from build123d import *

# Parameters (mm, degrees)
F0_R           = 10
F0_R_2         = 6.3
F1_DEPTH       = 6
F2_DEPTH       = 15
F4_R           = 1
F1_FACE_R      = 10
F7_D           = 4.3
F7_CBORE_D     = 8
F7_CBORE_DEPTH = 4.2
F8_D           = 3.2
F8_DEPTH       = 8
F8_START       = 6
F8_TIP         = 0.9613769904


with BuildPart() as f1:
    # F0 (on Top) → F1 (new body)
    with BuildSketch(Plane.XY):
        Circle(F0_R)
        Circle(F0_R_2, mode=Mode.SUBTRACT)
        Circle(F0_R_2)
    extrude(amount=F1_DEPTH)

    # F0 (on Top) → F2 (join)
    with BuildSketch(Plane.XY):
        Circle(F0_R)
        Circle(F0_R_2, mode=Mode.SUBTRACT)
    extrude(amount=-F2_DEPTH)

    # F7 (through all)
    with Locations(Plane(origin=(0, 0, 0), x_dir=(1, 0, 0), z_dir=(0, 0, -1))):
        with Locations((0, 0)):
            CounterBoreHole(F7_D / 2, F7_CBORE_D / 2, F7_CBORE_DEPTH)


with BuildPart() as f5:
    # F4 (on offset) → F5 section 0
    with BuildSketch(Plane.XY.offset(16)):
        Circle(F4_R)
    # F1_face (on face) → F5 section 1
    with BuildSketch(Plane.XY.offset(6)):
        Circle(F1_FACE_R)
    loft()

    # F8
    # its depths count from where the whole tool has entered the part; down to there all is cleared
    with Locations(Plane(origin=(0, 0, 0), x_dir=(1, 0, 0), z_dir=(0, 0, -1)).offset(-F8_START)):
        with Locations((0, 0)):
            Hole(F8_D / 2, depth=F8_DEPTH)
            with Locations((0, 0, -(F8_DEPTH + F8_TIP / 2))):  # 118° drill point
                Cone(0, F8_D / 2, F8_TIP, mode=Mode.SUBTRACT)


solid = f1.part
Can you work these out from the model? Positions are in its coordinate system, mm. A direction names the side the tool comes from. Give positions to 0.01 mm unless a question says otherwise; leave off trailing zeros. Loops run counter-clockwise (first coordinate to the right, second up) from the corner with the lowest first, then second, coordinate; pieces in that order, holes last. Notation, with made-up numbers: (-27, 10) -> (23, 10) arc R9 ccw to (23, 27) -> close; hole circle Ø2 at (28.5, 86.25). An arc over 180 degrees is marked (long way). Write item = value, one per line.
1) Suppose I cut it at C-C on x = 2.75. Write out the boundary of the cut face in (y, z).
Check result:
outline = (-9.61, -15) -> (-5.67, -15) -> (-5.67, 0) -> (-2.9, 0) -> (-2.9, 4.2) -> (2.9, 4.2) -> (2.9, 0) -> (5.67, 0) -> (5.67, -15) -> (9.61, -15) -> (9.61, 6) -> (-9.61, 6) -> close
2) Thinking about a two-plate mould opening in Y: for faces 3 (the flat face through (4.1, -1.3, 0)), 4 (the cylindrical face through (-2.17, -9.76, -4.35)), 5 (the flat face through (-0.1, 2.4, 6)), which applies, released by +Y, released by -Y, zero draft, split by the parting line, or undercut?
Check result:
face_3 = undercut
face_4 = split by the parting line
face_5 = zero draft
3) For faces 1 (the cylindrical face through (2.15, -0.09, 5.11)), 2 (the flat face through (2, 2, 4.2)), which set-ups out of +Z, -Z, +X, -X, +Y, -Y let a thin tool reach every point of the face, with its end or its side?
Check result:
face_1 = +Z, -Z
face_2 = -Z
4) I need wall thicknesses on L1, parallel to Y at x = 0, z = -5.75; L2, parallel to Y at x = 0, z = 1.9; L3, parallel to Z at x = -2.25, y = 3.75. Which ranges of each line are inside material? Lowest first, please. Write a range as from..to.
Check result:
L1 = -10..-6.3, 6.3..10
L2 = -10..-4, 4..10
L3 = 0..6
5) Suppose I cut it at A-A on y = 0. Write out the boundary of the cut face in (x, z).
Check result:
outline = (-10, -15) -> (-6.3, -15) -> (-6.3, 0) -> (-4, 0) -> (-4, 4.2) -> (-2.15, 4.2) -> (-2.15, 6) -> (-10, 6) -> close; (2.15, 4.2) -> (4, 4.2) -> (4, 0) -> (6.3, 0) -> (6.3, -15) -> (10, -15) -> (10, 6) -> (2.15, 6) -> close
6) Suppose I cut it at D-D on z = -4.25. Write out the boundary of the cut face in (x, y).
Check result:
outline = circle Ø20 at (0, 0); hole circle Ø12.6 at (0, 0)
7) Will these pins go through, and if not, where does the flat tip stop? pin 1 (6.5 mm diameter, centred on x = 2, y = 1.5, fed in from -Z); pin 2 (1 mm diameter, centred on x = 2.5, z = -11.5, fed in from +Y); pin 3 (3 mm diameter, centred on y = -4.5, z = -8.5, fed in from +X); pin 4 (4 mm diameter, centred on x = 0, y = 0, fed in from +Z).
Check result:
pin_1 = 0
pin_2 = 9.8
pin_3 = 9.54
pin_4 = through
